For this review, use the dimensioned drawing (mm, ordinates from the lowest corner) and the shaded views. Give positions to 0.01 mm unless a question says otherwise; leave off trailing zeros. Order: outer loops, then holes, each group sorted by start corner. A loop starts at its lowest first (then second) coordinate and runs counter-clockwise, first axis right, second up. Notation, with made-up numbers: (1, 68.25) - (22, 68.25) arc R19 ccw to (22, 91.25) - close; hole circle Ø9 at (-22.75, 28). An arc over 180 degrees is marked (long way). One line per item, written item: value.
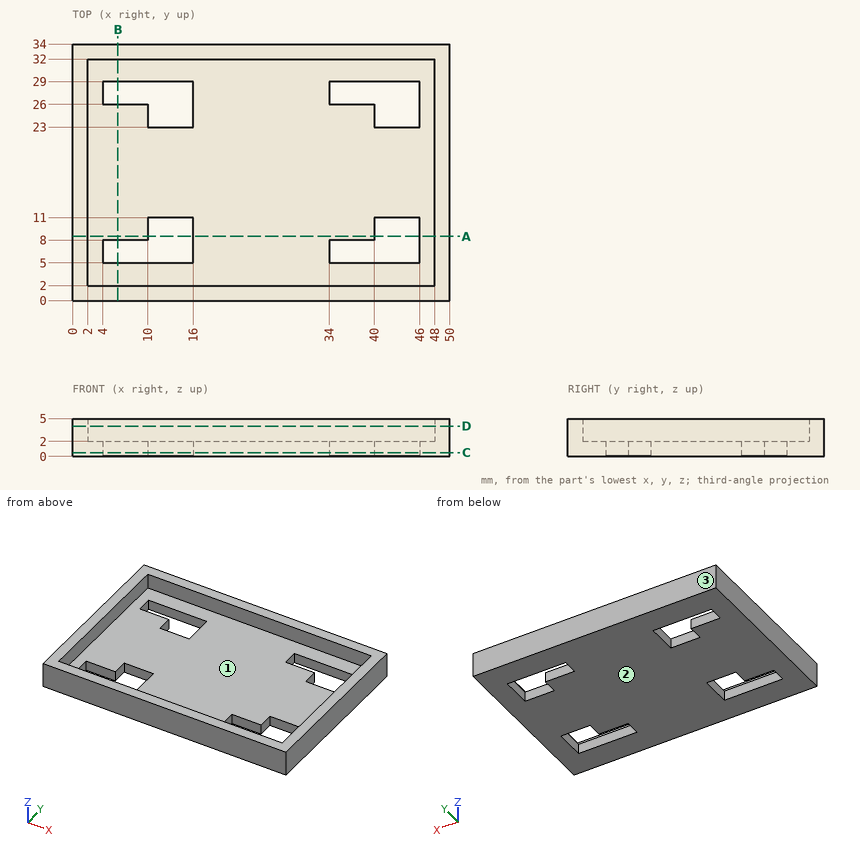
(1) Draft analysis for pull direction Y (two halves, no side actions). For the marked faces 1, 2 and 3, state which applies: pulls with the +Y half, pulls with the -Y half, needs draft (parallel to the pull), parting line crosses it, or undercut.
Answers below:
face 1: undercut
face 2: needs draft
face 3: pulls with the +Y half
(2) Take a section at D-D (z = 4). Write out the cut boundary in (x, y).
Answers below:
outline: (0, 0) - (50, 0) - (50, 34) - (0, 34) - close; hole (2, 2) - (48, 2) - (48, 32) - (2, 32) - close
(3) Take a section at B-B (x = 6). Write out the cut boundary in (y, z), then the cut area to 3 significant figures.
Answers below:
outline: (0, 0) - (5, 0) - (5, 2) - (2, 2) - (2, 5) - (0, 5) - close; (8, 0) - (26, 0) - (26, 2) - (8, 2) - close; (29, 0) - (34, 0) - (34, 5) - (32, 5) - (32, 2) - (29, 2) - close
area: 68.0 mm^2
(4) Take a section at C-C (z = 0.5). Write out the cut boundary in (x, y), then the cut area to 3 significant figures.
Answers below:
outline: (0, 0) - (50, 0) - (50, 34) - (0, 34) - close; hole (4, 5) - (16, 5) - (16, 11) - (10, 11) - (10, 8) - (4, 8) - close; hole (4, 26) - (10, 26) - (10, 23) - (16, 23) - (16, 29) - (4, 29) - close; hole (34, 5) - (46, 5) - (46, 11) - (40, 11) - (40, 8) - (34, 8) - close; hole (34, 26) - (40, 26) - (40, 23) - (46, 23) - (46, 29) - (34, 29) - close
area: 1,480 mm^2
(5) For P1, Ø2, axis at x = 21, y = 13, coming from the +Z side, flat-tipped, find the tip position at first contact; note if it passes through.
Answers below:
P1: stops at z = 2
(6) Wall thickness on line 1 (X direction, y = 11, z = 4.45); line 2 (Y direction, x = 44, z = 0.85); line 3 (Y direction, x = 46, z = 2.2): over which ranges is each line inside the solid? List them lowest first. Write a range as from..to.
Answers below:
line 1: x = 0..2, 48..50
line 2: y = 0..5, 11..23, 29..34
line 3: y = 0..2, 32..34
(7) Take a section at A-A (y = 8.5). Write out the cut boundary in (x, z), then the cut area to 3 significant figures.
Answers below:
outline: (0, 0) - (10, 0) - (10, 2) - (2, 2) - (2, 5) - (0, 5) - close; (16, 0) - (40, 0) - (40, 2) - (16, 2) - close; (46, 0) - (50, 0) - (50, 5) - (48, 5) - (48, 2) - (46, 2) - close
area: 88.0 mm^2
